For this review, take the finished solid that the model builds, in its own axes (mm). Face numbers are marked on the shaded views. Round coordinates to 2 decimals unless told otherwise and drop trailing zeros. Write each loop counter-clockwise with the first axis right and the second up, starting at its lowest first coordinate (ties: lowest second). Pieces come first, ordered by that corner, then holes. Notation, with made-up numbers: (-34, -33.5) - (13, -33.5) arc R22 ccw to (13, -23.5) - close; hole circle Ø4 at (79.5, -24.5). An arc over 180 degrees is marked (long way). One line per item, written item: value. Start each with the question number.
Q1. For probe 1 along Z at (x, y) = (-9, 23.5); probe 2 along X at (y, z) = (-6, -17); probe 3 along Y at (x, z) = (13.5, -9), list the stretches that pass through material, from the lowest coordinate up.
Q2. Add section D-D on x = 0. Write out the cut boundary in (y, z).
Q3. Mouldability with a two-part tool opening along X and no side actions: class the marked faces 1, 2 and 3 as +X half, -X half, draft (parallel to the pull), parting line (faces both ways), or undercut.
Q4. Add section B-B on y = 23. Write out the cut boundary in (x, z), and give its area (3 significant figures).
Q5. Add section A-A on z = -36. Write out the cut boundary in (x, y), and give its area (3 significant figures).
Q6. Clearance check with flat-ended pins moving along their axes: pin 1 Ø2.5 at (y, z) = (40, -26.5) entering from -X; pin 2 Ø15 at (x, y) = (-7.5, 19.5) entering from +Z; pin 3 Ø10 at (y, z) = (15, -1) entering from +X. State where each tip first meets the part, or that it passes through.
Q7. Add section C-C on z = 2.5. Give the number of separate pieces and of enclosed holes in the cut face, and give its area (3 significant figures).
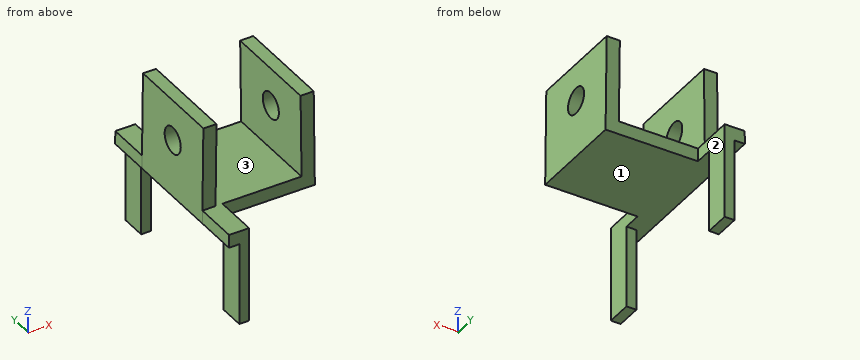
```python
from build123d import *

# Parameters (mm, degrees)
BOSS_EXTRUDE1_DEPTH      = 30
SKETCH3_R                = 4
CUT_EXTRUDE1_DEPTH       = 40
SKETCH4_W                = 3
SKETCH4_H                = 41
BOSS_EXTRUDE2_DEPTH      = 4
BOSS_EXTRUDE3_DEPTH      = 25
BOSS_EXTRUDE3_DEPTH_BACK = 4
SKETCH5_W                = 3
SKETCH5_H                = 7.75
BOSS_EXTRUDE4_REACH      = 69.734
SKETCH6_W                = 4
SKETCH6_H                = 56.5


with BuildPart() as part:
    # Sketch1 → Boss-Extrude1 (new body)
    with BuildSketch(Plane(origin=(0, 0, 0), x_dir=(1, 0, 0), z_dir=(0, 1, 0))):
        Polygon((-12.8, -12.8), (-13.1, 12.8), (13.1, 12.8), (12.8, -12.6), (16.799721029, -12.6472408), (17.147523085, 16.8), (-17.147149649, 16.8), (-16.79972537, -12.846871782), align=None)
    extrude(amount=BOSS_EXTRUDE1_DEPTH)

    # Sketch3 → Cut-Extrude1 (cut)
    with BuildSketch(Plane(origin=(16.946733814, 0, 0.200158273), x_dir=(0.011810199887684227, 0, -0.9999302571572745), z_dir=(0.9999302571572745, 0, 0.011810199887684227))):
        with Locations(Location((-0.747950682, 15, 0), (0, 0, 180))):
            Circle(SKETCH3_R)
    extrude(amount=-CUT_EXTRUDE1_DEPTH, mode=Mode.SUBTRACT)

    # Sketch4 → Boss-Extrude2 (add)
    with BuildSketch(Plane(origin=(0, 0, -16.8), x_dir=(-1, 0, 0), z_dir=(0, 0, -1))):
        with Locations((12.499813282, 15)):
            Rectangle(SKETCH4_W, SKETCH4_H)
    extrude(amount=-BOSS_EXTRUDE2_DEPTH)

    # Sketch5 → Boss-Extrude3 (add, two sides: drawn at the far end of the back side and taken through both)
    with BuildSketch(Plane(origin=(0, 0, -16.8), x_dir=(-1, 0, 0), z_dir=(0, 0, -1)).offset(-BOSS_EXTRUDE3_DEPTH_BACK)):
        with Locations((12.499813282, 39.375)):
            Rectangle(SKETCH5_W, SKETCH5_H)
        with Locations((12.499813282, -9.375)):
            Rectangle(SKETCH5_W, SKETCH5_H)
    extrude(amount=BOSS_EXTRUDE3_DEPTH + BOSS_EXTRUDE3_DEPTH_BACK)

    # Boss-Extrude4: up to this plane
    boss_extrude4_end = Plane(origin=(-16.79972537, 30, 12.846871782), z_dir=(0.9999313425206403, 0, -0.01171794542016394))
    # Sketch6 → Boss-Extrude4 (add, up to the surface)
    with BuildSketch(Plane.ZY.offset(13.999813282), mode=Mode.PRIVATE) as boss_extrude4_sk1:
        with Locations((-14.8, 15)):
            Rectangle(SKETCH6_W, SKETCH6_H)
    boss_extrude4_tool1 = split(extrude(boss_extrude4_sk1.sketch, amount=BOSS_EXTRUDE4_REACH, mode=Mode.PRIVATE), bisect_by=boss_extrude4_end, keep=Keep.BOTH, mode=Mode.PRIVATE)
    add(boss_extrude4_tool1.solids().sort_by_distance((-13.999813, 15, -14.8))[0])


solid = part.part
```
Result set:
1. probe 1: z = -16.8 to -12.8
1. probe 2: x = -14 to -11
1. probe 3: y = 0 to 30
2. outline: (0, -16.8) - (30, -16.8) - (30, -12.8) - (0, -12.8) - close
3. face 1: draft
3. face 2: +X half
3. face 3: undercut
4. outline: (-17.15, -16.8) - (17.15, -16.8) - (16.8, 12.65) - (12.8, 12.6) - (13.1, -12.8) - (-13.1, -12.8) - (-12.8, 12.8) - (-16.8, 12.85) - close
4. area: 341 mm^2
5. outline: (-14, -13.25) - (-11, -13.25) - (-11, -5.5) - (-14, -5.5) - close; (-14, 35.5) - (-11, 35.5) - (-11, 43.25) - (-14, 43.25) - close
5. area: 46.5 mm^2
6. pin 1: stops at x = -14
6. pin 2: stops at z = 12.83
6. pin 3: stops at x = 17.02
7. separate pieces: 4
7. enclosed holes: 0
7. area: 183 mm^2
